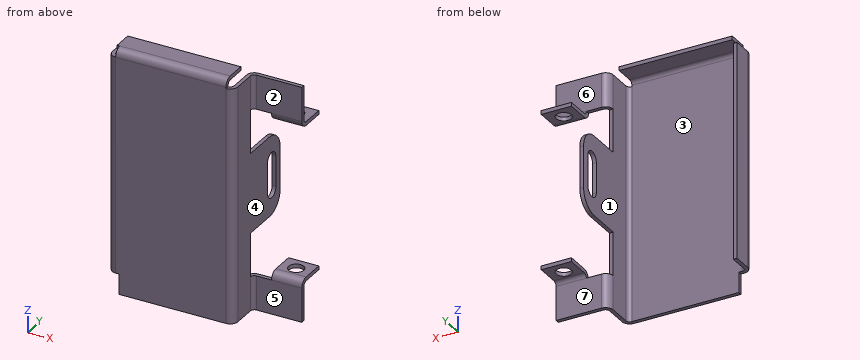
```python
from build123d import *

# Parameters (mm, degrees)
Z_KLADN_PLECH1_DEPTH     = 62
LEM_Z_HRANY1_DEPTH       = 29.17
LEM_START                = 1
LEM_Z_HRANY1_PROFILE_W   = 29.89
LEM_Z_HRANY1_PROFILE_H   = 5
LEM_Z_HRANY1_FLAT_DEPTH  = 1
LEM_Z_HRANY2_DEPTH       = 57
SKICA12_W                = 5.36
SKICA12_H                = 1
ODEBRAT_VYSUNUT_M1_DEPTH = 0.9
OU_KO2_DEPTH             = 1
LEM_Z_HRANY3_DEPTH       = 9
LEM_Z_HRANY4_DEPTH       = 8
ODEBRAT_VYSUNUT_M2_REACH = 73.386
SKICA25_R                = 2
LEM_Z_HRANY5_DEPTH       = 9


# Sheet-metal steps are written as plain solids
with BuildPart() as part:
    # Skica1 → Základní plech1 (new body)
    with BuildSketch(Plane.XY):
        with BuildLine():
            Line((0, 0), (29.17, 0))
            ThreePointArc((29.17, 0), (29.877106781, 0.292893219), (30.17, 1))
            Line((30.17, 1), (30.17, 7))
            Line((30.17, 7), (31.17, 7))
            Line((31.17, 7), (31.17, 1))
            ThreePointArc((31.17, 1), (30.584213562, -0.414213562), (29.17, -1))
            Line((29.17, -1), (0, -1))
            Line((0, -1), (0, 0))
        make_face()
    extrude(amount=Z_KLADN_PLECH1_DEPTH)

    # Lem z hrany1 bend section (across the edge) → Lem z hrany1 (add)
    with BuildSketch(Plane(origin=(0, 0, 63.36), x_dir=(0, 0, -1), z_dir=(1, 0, 0))):
        with BuildLine():
            Line((-1, 1), (0, 1))
            ThreePointArc((0, 1), (0.292893219, 0.292893219), (1, 0))
            Line((1, 0), (1.36, 0))
            Line((1.36, 0), (1.36, -1))
            Line((1.36, -1), (1, -1))
            ThreePointArc((1, -1), (-0.414213562, -0.414213562), (-1, 1))
        make_face()
    extrude(amount=LEM_Z_HRANY1_DEPTH)

    # Lem z hrany1 profile (on flange) → Lem z hrany1 flat (add)
    with BuildSketch(Plane.XY.offset(63.36).offset(LEM_START)):
        with Locations((14.225, 3.5)):
            Rectangle(LEM_Z_HRANY1_PROFILE_W, LEM_Z_HRANY1_PROFILE_H)
    extrude(amount=-LEM_Z_HRANY1_FLAT_DEPTH)

    # Lem z hrany2 section (across the edge) → Lem z hrany2 (add)
    with BuildSketch(Plane(origin=(-1, 0, 5.36), x_dir=(1, 0, 0), z_dir=(0, 0, 1))):
        with BuildLine():
            Line((-1, 1), (-1, 6))
            Line((-1, 6), (0, 6))
            Line((0, 6), (0, 1))
            ThreePointArc((0, 1), (0.292893219, 0.292893219), (1, 0))
            Line((1, 0), (1, -1))
            ThreePointArc((1, -1), (-0.414213562, -0.414213562), (-1, 1))
        make_face()
    extrude(amount=LEM_Z_HRANY2_DEPTH)

    # Skica12 → Odebrat vysunutím1 (cut)
    with BuildSketch(Plane.ZY):
        with Locations((2.68, -0.5)):
            Rectangle(SKICA12_W, SKICA12_H)
    extrude(amount=-ODEBRAT_VYSUNUT_M1_DEPTH, mode=Mode.SUBTRACT)

    # Skica13 → Ouško2 (add)
    with BuildSketch(Plane.ZY.offset(-30.17)):
        with BuildLine():
            Line((20.5, 7), (20.5, 16))
            ThreePointArc((20.5, 16), (21.964466094, 19.535533906), (25.5, 21))
            Line((25.5, 21), (36.5, 21))
            ThreePointArc((36.5, 21), (40.035533906, 19.535533906), (41.5, 16))
            Line((41.5, 16), (41.5, 7))
            Line((41.5, 7), (20.5, 7))
        make_face()
        with BuildLine():
            Line((27, 19), (35, 19))
            ThreePointArc((35, 19), (37, 17), (35, 15))
            Line((35, 15), (27, 15))
            ThreePointArc((27, 15), (25, 17), (27, 19))
        make_face(mode=Mode.SUBTRACT)
    extrude(amount=-OU_KO2_DEPTH)

    # Lem z hrany3 section (across the edge) → Lem z hrany3 (add)
    with BuildSketch(Plane(origin=(31.17, 8, 53), x_dir=(0, -1, 0), z_dir=(0, 0, 1))):
        with BuildLine():
            Line((-1, 1), (-1, 13))
            Line((-1, 13), (0, 13))
            Line((0, 13), (0, 1))
            ThreePointArc((0, 1), (0.292893219, 0.292893219), (1, 0))
            Line((1, 0), (1, -1))
            ThreePointArc((1, -1), (-0.414213562, -0.414213562), (-1, 1))
        make_face()
    extrude(amount=LEM_Z_HRANY3_DEPTH)

    # Lem z hrany4 section (across the edge) → Lem z hrany4 (add)
    with BuildSketch(Plane(origin=(44.17, 9, 52), x_dir=(0, 0, 1), z_dir=(-1, 0, 0))):
        with BuildLine():
            Line((-1, 1), (-1, 7))
            Line((-1, 7), (0, 7))
            Line((0, 7), (0, 1))
            ThreePointArc((0, 1), (0.292893219, 0.292893219), (1, 0))
            Line((1, 0), (1, -1))
            ThreePointArc((1, -1), (-0.414213562, -0.414213562), (-1, 1))
        make_face()
    lem_z_hrany4 = extrude(amount=LEM_Z_HRANY4_DEPTH)

    # Skica25 → Odebrat vysunutím2 (cut, up to next)
    with BuildSketch(Plane.XY.offset(52), mode=Mode.PRIVATE) as odebrat_vysunut_m2_sk1:
        with Locations((40.17, 12.5)):
            Circle(SKICA25_R)
    odebrat_vysunut_m2_tool1 = extrude(odebrat_vysunut_m2_sk1.sketch, amount=-ODEBRAT_VYSUNUT_M2_REACH, mode=Mode.PRIVATE) & part.part
    odebrat_vysunut_m2 = odebrat_vysunut_m2_tool1.solids().sort_by_distance((40.17, 12.5, 52))[0]
    add(odebrat_vysunut_m2, mode=Mode.SUBTRACT)

    # Lem z hrany5 section (across the edge) → Lem z hrany5 (add)
    with BuildSketch(Plane(origin=(31.17, 8, 0), x_dir=(0, -1, 0), z_dir=(0, 0, 1))):
        with BuildLine():
            Line((-1, 1), (-1, 13))
            Line((-1, 13), (0, 13))
            Line((0, 13), (0, 1))
            ThreePointArc((0, 1), (0.292893219, 0.292893219), (1, 0))
            Line((1, 0), (1, -1))
            ThreePointArc((1, -1), (-0.414213562, -0.414213562), (-1, 1))
        make_face()
    extrude(amount=LEM_Z_HRANY5_DEPTH)

    # Zrcadlit1: Lem z hrany4, Odebrat vysunutím2 across plane
    add(lem_z_hrany4.mirror(Plane.XY.offset(31)))
    add(odebrat_vysunut_m2.mirror(Plane.XY.offset(31)), mode=Mode.SUBTRACT)


solid = part.part
```
Here's how the part is built. I have some questions about the finished solid (model axes, mm). Face numbers are marked on the shaded views. A direction names the side the tool comes from. Round coordinates to 2 decimals unless told otherwise and drop trailing zeros. Write each loop counter-clockwise with the first axis right and the second up, starting at its lowest first coordinate (ties: lowest second). Pieces come first, ordered by that corner, then holes. Notation, with made-up numbers: M 40,29.5 L 45,29.5 A38 cw 45,68.5 Z; hole C 24,17 d2. An arc over 180 degrees is marked long. Answer as CSV lines item,"result". Start each with the question number.
1. Suppose I cut it at D-D on z = 50. Write out the boundary of the cut face in (x, y), then the cut area to 3 significant figures.
2. I need wall thicknesses on probe 1 along X at (y, z) = (1.25, 19); probe 2 along Y at (x, z) = (9.5, 18.5); probe 3 along Z at (x, y) = (2, 1.25). Which ranges of each line are inside material? Lowest first, please.
3. Thinking about a two-plate mould opening in X: for the marked faces 1, 2, 3 and 4, which applies, released by +X, released by -X, zero draft, split by the parting line, or undercut?
4. On a 3-axis mill with a long thin cutter (end or side, diameter ignored), from which of +Z, -Z, +X, -X, +Y, -Y can I reach the whole of each face in a straight line? I mean the marked faces 5, 6 and 7. Say none if no direction works.
5. Suppose I cut it at C-C on x = 20.5. Write out the boundary of the cut face in (y, z).
6. Suppose I cut it at A-A on x = 40.17. Write out the boundary of the cut face in (y, z).
7. I'm going to push flat-ended pins straight in: pin 1 Ø5 at (x, y) = (41.5, 13) entering from +Z; pin 2 Ø1.1 at (x, z) = (39.5, 51.5) entering from +Y; pin 3 Ø2 at (y, z) = (11.5, 9.5) entering from -X. Where does each tip first touch, or does it pass through?
8. Suppose I cut it at B-B on y = 12.5. Write out the boundary of the cut face in (x, z).
Check result:
1,outline,"M -2,1 A2 ccw 0,-1 L 29.17,-1 A2 ccw 31.17,1 L 31.17,7 L 30.17,7 L 30.17,1 A1 cw 29.17,0 L 0,0 A1 cw -1,1 L -1,6 L -2,6 Z"
1,area,"44.9 mm2"
2,probe 1,"x = -2 to -1, 30.17 to 31.17"
2,probe 2,"y = -1 to 0"
2,probe 3,"z = 63.36 to 64.36"
3,face 1,"undercut"
3,face 2,"zero draft"
3,face 3,"undercut"
3,face 4,"released by +X"
4,face 5,"+Z, -Z, +X, -Y"
4,face 6,"+Z, +X, -X, +Y"
4,face 7,"-Z, +X, -X, +Y"
5,outline,"M -1,0 L 0,0 L 0,62.36 A1 cw 1,63.36 L 6,63.36 L 6,64.36 L 1,64.36 A2 ccw -1,62.36 Z"
6,outline,"M 8,0 L 9,0 L 9,9 A1 cw 10,10 L 10.5,10 L 10.5,11 L 10,11 A2 ccw 8,9 Z; M 8,53 A2 ccw 10,51 L 10.5,51 L 10.5,52 L 10,52 A1 cw 9,53 L 9,62 L 8,62 Z; M 14.5,10 L 16,10 L 16,11 L 14.5,11 Z; M 14.5,51 L 16,51 L 16,52 L 14.5,52 Z"
7,pin 1,"stops at z = 52"
7,pin 2,"stops at y = 16"
7,pin 3,"stops at x = 36.17"
8,outline,"M 30.17,20.5 L 31.17,20.5 L 31.17,41.5 L 30.17,41.5 Z; M 36.17,10 L 38.17,10 L 38.17,11 L 36.17,11 Z; M 36.17,51 L 38.17,51 L 38.17,52 L 36.17,52 Z; M 42.17,10 L 44.17,10 L 44.17,11 L 42.17,11 Z; M 42.17,51 L 44.17,51 L 44.17,52 L 42.17,52 Z"
